Geometry: final body of the model. Coordinates: model frame, mm. A direction names the side the tool comes from. Round coordinates to 2 decimals unless told otherwise and drop trailing zeros. Order: outer loops, then holes, each group sorted by start corner. A loop starts at its lowest first (then second) coordinate and runs counter-clockwise, first axis right, second up. Notation, with made-up numbers: (18.25, 32.25) - (74.25, 32.25) arc R10 ccw to (74.25, 40.25) - close; hole circle Ø2 at (84, -7.5). An arc over 180 degrees is marked (long way). Put each result on its own line as item: value. Start each with the question number.
(1) Pin query (flat end, axial travel): P1, Ø1.2, axis at y = 1.5, z = 37, coming from the +X side; P2, Ø4, axis at x = 15, y = 7, coming from the +Z side; P3, Ø2, axis at x = 14, y = 6.5, coming from the +Z side; P4, Ø3, axis at x = 6.5, z = 23, coming from the -Y side. Return the tip coordinate at first contact, or that it passes through.
(2) Section A-A (z = 109.2). Output: boundary loops of the cut face in (x, y), and give its area (4 significant figures).
(3) Section C-C (x = 3.75). Output: boundary loops of the cut face in (y, z).
(4) Section B-B (x = 14.5). Output: boundary loops of the cut face in (y, z).
(5) Access query for faces 5 (the face through (3, 3, 0)), 6 (the face through (7, 4, 52)), 7 (the face through (15, 2, 0)). Directions: +Z, -Z, +X, -X, +Y, -Y. A direction counts if a zero-diameter tool reaches every point of the face in a straight line with its end or side. Return the directions, or none.
(6) Pull-direction query (Y, two-part tool) for faces 1 (the face through (9.86, 4.77, 110.9)), 2 (the face through (10, 2, -7.9)), 3 (the face through (10.14, 4.975, -0.359)), 4 (the face through (9.86, 6.386, -3.979)); classes: released by +Y, released by -Y, zero draft, split by the parting line, or undercut.
(7) Material intervals for L1, parallel to Z at x = 6, y = 3.5; L2, parallel to Y at x = 6, z = 109.2; L3, parallel to Z at x = 17.75, y = 6, sorted ascending. Write a range as [from, to].
(8) Section D-D (z = 28.5). Output: boundary loops of the cut face in (x, y).
from build123d import *

# Parameters (mm, degrees)
RESSALTO_EXTRUS_O1_DEPTH      = 100
ESBO_O3_W                     = 10
ESBO_O3_H                     = 4
RESSALTO_EXTRUS_O2_DEPTH      = 5
ESBO_O4_R                     = 1.7
RESSALTO_EXTRUS_O3_DEPTH      = 10
RESSALTO_EXTRUS_O3_DEPTH_BACK = 10


with BuildPart() as part:
    # Esboço1 → Ressalto-extrusão1 (new body)
    with BuildSketch(Plane.XY):
        Polygon((0, 0), (0, 2), (5, 2), (5, 4), (10, 4), (10, 0), align=None)
    extrude(amount=RESSALTO_EXTRUS_O1_DEPTH)

    # Esboço3 → Ressalto-extrusão2 (add)
    with BuildSketch(Plane.XY.offset(100)):
        with Locations((5, 2)):
            Rectangle(ESBO_O3_W, ESBO_O3_H)
    extrude(amount=RESSALTO_EXTRUS_O2_DEPTH)

    # Esboço4 → Ressalto-extrusão3 (add, two sides)
    with BuildSketch(Plane(origin=(10, 0, 0), x_dir=(0, 0, -1), z_dir=(1, 0, 0))) as ressalto_extrus_o3_sk:
        with BuildLine():
            Line((-112.9, 4.7), (-112.9, 0))
            Line((-112.9, 0), (-105, 0))
            Line((-105, 0), (-105, 4))
            Line((-105, 4), (-105.72755275, 5.977540643))
            ThreePointArc((-105.72755275, 5.977540643), (-109.848824003, 8.342667623), (-112.9, 4.7))
        make_face()
        with Locations((-109.2, 4.7)):
            Circle(ESBO_O4_R, mode=Mode.SUBTRACT)
        with BuildLine():
            Line((7.9, 0), (0, 0))
            Line((0, 0), (0, 4))
            Line((0, 4), (0.72755275, 5.977540643))
            ThreePointArc((0.72755275, 5.977540643), (4.848824003, 8.342667623), (7.9, 4.7))
            Line((7.9, 4.7), (7.9, 0))
        make_face()
        with Locations((4.2, 4.7)):
            Circle(ESBO_O4_R, mode=Mode.SUBTRACT)
    extrude(amount=RESSALTO_EXTRUS_O3_DEPTH)
    extrude(ressalto_extrus_o3_sk.sketch, amount=-RESSALTO_EXTRUS_O3_DEPTH_BACK)


solid = part.part
Checks:
1. P1: stops at x = 10
1. P2: stops at z = 112.89
1. P3: stops at z = 112.81
1. P4: stops at y = 0
2. outline: (0, 0) - (20, 0) - (20, 3) - (0, 3) - close; (0, 6.4) - (20, 6.4) - (20, 8.4) - (0, 8.4) - close
2. area: 100.0 mm²
3. outline: (0, -7.9) - (4.7, -7.9) arc R3.7 ccw to (5.98, -0.73) - (4, 0) - (2, 0) - (2, 100) - (4, 100) - (4, 105) - (5.98, 105.73) arc R3.7 ccw to (4.7, 112.9) - (0, 112.9) - close; hole circle Ø3.4 at (4.7, -4.2); hole circle Ø3.4 at (4.7, 109.2)
4. outline: (0, -7.9) - (4.7, -7.9) arc R3.7 ccw to (5.98, -0.73) - (4, 0) - (0, 0) - close; (0, 105) - (4, 105) - (5.98, 105.73) arc R3.7 ccw to (4.7, 112.9) - (0, 112.9) - close; hole circle Ø3.4 at (4.7, -4.2); hole circle Ø3.4 at (4.7, 109.2)
5. face 5: -X, +Y
5. face 6: +X, -X, +Y
5. face 7: +X, +Y, -Y
6. face 1: undercut
6. face 2: zero draft
6. face 3: released by +Y
6. face 4: undercut
7. L1: z = [-7.9, -5.4], [-3, 108], [110.4, 112.9]
7. L2: y = [0, 3], [6.4, 8.4]
7. L3: z = [-7.66, -5.3], [-3.1, -0.74], [105.74, 108.1], [110.3, 112.66]
8. outline: (0, 0) - (10, 0) - (10, 4) - (5, 4) - (5, 2) - (0, 2) - close
